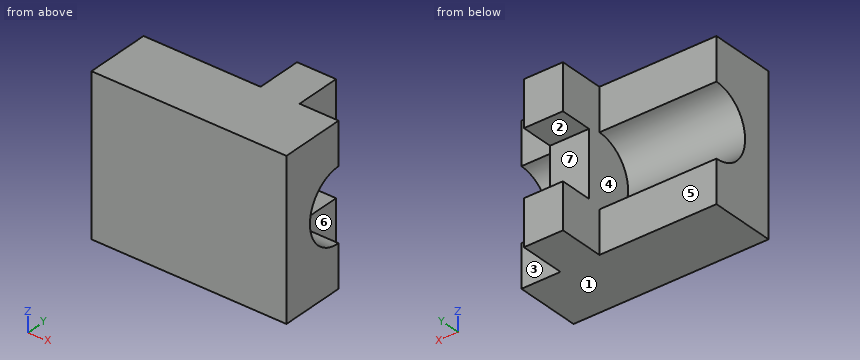
```python
from build123d import *

# Parameters (mm, degrees)
EXTRUDE_1_DEPTH = 75
EXTRUDE_2_DEPTH = 30


with BuildPart() as part:
    # Эскиз1 → Бобышка-Вытянуть1 (new, symmetric)
    with BuildSketch(Plane(origin=(0, 0, 0), x_dir=(0, 0, -1), z_dir=(1, 0, 0))):
        with BuildLine():
            Line((-60, 25), (-60, -25))
            Line((-60, -25), (60, -25))
            Line((60, -25), (60, 25))
            Line((60, 25), (27.5, 25))
            ThreePointArc((27.5, 25), (0, -2.5), (-27.5, 25))
            Line((-27.5, 25), (-60, 25))
        make_face()
    extrude(amount=EXTRUDE_1_DEPTH, both=True)

    # Эскиз2 → Бобышка-Вытянуть2 (add)
    with BuildSketch(Plane(origin=(45, 0, 0), x_dir=(0, 0, -1), z_dir=(1, 0, 0))):
        Polygon((-60, -25), (60, -25), (60, 60), (25, 60), (25, 35), (-25, 35), (-25, 60), (-60, 60), align=None)
    extrude(amount=-EXTRUDE_2_DEPTH)


solid = part.part
```
Verification items for the finished model (mm, model axes). Face numbers are marked on the shaded views. A direction names the side the tool comes from. Coordinates: 2 decimals unless noted, no trailing zeros. Loops run counter-clockwise (first coordinate to the right, second up) from the corner with the lowest first, then second, coordinate; pieces in that order, holes last. Notation, with made-up numbers: (0.25, -25.75) -> (51.25, -25.75) arc R27 ccw to (51.25, -6.75) -> close; hole circle Ø8 at (11.5, -17). An arc over 180 degrees is marked (long way). Answer in a Markdown table with one row per item.
1) Section check C-C (z = 0). Record the cut outline in (x, y), and give its area (3 significant figures).
The answers:
| item | result |
|---|---|
| outline | (-75, -25) -> (75, -25) -> (75, -2.5) -> (45, -2.5) -> (45, 35) -> (15, 35) -> (15, -2.5) -> (-75, -2.5) -> close |
| area | 4,500 mm2 |
2) Draft check along Z on the marked faces 1, 2 and 3. Enter one of: released by +Z, released by -Z, zero draft, split by the parting line, or undercut.
The answers:
| item | result |
|---|---|
| face 1 | released by -Z |
| face 2 | undercut |
| face 3 | zero draft |
3) Depth check by flat-ended pin: P1, Ø12, axis at y = 31.5, z = -43.5, coming from the +X side; P2, Ø10, axis at x = -37.5, z = -45, coming from the +Y side; P3, Ø9, axis at x = 24, z = -1.5, coming from the +Y side. Enter the tip coordinate at first touch or a pass-through.
The answers:
| item | result |
|---|---|
| P1 | stops at x = 45 |
| P2 | stops at y = 25 |
| P3 | stops at y = 35 |
4) Section check D-D (x = -11). Record the cut outline in (y, z), and give its area (3 significant figures).
The answers:
| item | result |
|---|---|
| outline | (-25, -60) -> (25, -60) -> (25, -27.5) arc R27.5 cw to (25, 27.5) -> (25, 60) -> (-25, 60) -> close |
| area | 4,810 mm2 |
5) Section check A-A (y = 45). Record the cut outline in (x, z).
The answers:
| item | result |
|---|---|
| outline | (15, -60) -> (45, -60) -> (45, -25) -> (15, -25) -> close; (15, 25) -> (45, 25) -> (45, 60) -> (15, 60) -> close |
6) Access from +Z, -Z, +X, -X, +Y, -Y to the whole of each face (thin tool, end or side, straight path). Record for the marked faces 4, 5, 6 and 7.
The answers:
| item | result |
|---|---|
| face 4 | -X, +Y |
| face 5 | +Z, -Z, -X, +Y |
| face 6 | +X, +Y |
| face 7 | +X, -X, +Y |
7) Section check B-B (x = 35.5). Record the cut outline in (y, z).
The answers:
| item | result |
|---|---|
| outline | (-25, -60) -> (60, -60) -> (60, -25) -> (35, -25) -> (35, 25) -> (60, 25) -> (60, 60) -> (-25, 60) -> close |
8) Scan lines: line 1 along X through (y, z) = (53.5, -26); line 2 along Y through (x, z) = (68, -50.5); line 3 along Z through (x, y) = (54.5, 10.5). Record each from-to range of solid material in increasing order. Write a range as from..to.
The answers:
| item | result |
|---|---|
| line 1 | x = 15..45 |
| line 2 | y = -25..25 |
| line 3 | z = -60..-23.37, 23.37..60 |
